from build123d import *

# Parameters (mm, degrees)
SKETCH2_W           = 15
SKETCH2_H           = 20
BOSS_EXTRUDE1_DEPTH = 9
SKETCH3_R           = 1.75
CUT_EXTRUDE1_DEPTH  = 18.400072003
SKETCH4_W           = 35
SKETCH4_H           = 15
BOSS_EXTRUDE2_DEPTH = 9
SKETCH5_R           = 1.75
CUT_EXTRUDE2_DEPTH  = 47.61728645


with BuildPart() as part:
    # Sketch2 → Boss-Extrude1 (new body)
    with BuildSketch(Plane(origin=(0, 0, 0), x_dir=(0, 0, -1), z_dir=(1, 0, 0))):
        with Locations((2.852361856, -0.704723711)):
            Rectangle(SKETCH2_W, SKETCH2_H)
    extrude(amount=BOSS_EXTRUDE1_DEPTH)

    # Sketch3 → Cut-Extrude1 (cut, through all)
    with BuildSketch(Plane(origin=(9, 0, 0), x_dir=(0, 0, -1), z_dir=(1, 0, 0))):
        with Locations((2.852361856, -5.704723711)):
            Circle(SKETCH3_R)
        with Locations((2.852361856, 4.295276289)):
            Circle(SKETCH3_R)
    extrude(amount=-CUT_EXTRUDE1_DEPTH, mode=Mode.SUBTRACT)

    # Sketch4 → Boss-Extrude2 (add)
    with BuildSketch(Plane(origin=(0, 9.295276289, 0), x_dir=(1, 0, 0), z_dir=(0, 1, 0))):
        with Locations((17.5, 2.852361856)):
            Rectangle(SKETCH4_W, SKETCH4_H)
    extrude(amount=BOSS_EXTRUDE2_DEPTH)

    # Sketch5 → Cut-Extrude2 (cut, through all)
    with BuildSketch(Plane(origin=(0, 18.295276289, 0), x_dir=(1, 0, 0), z_dir=(0, 1, 0))):
        with Locations(Location((12, 2.852361856, 0), (0, 0, 270))):
            Circle(SKETCH5_R)
        with Locations(Location((22, 2.852361856, 0), (0, 0, 270))):
            Circle(SKETCH5_R)
    extrude(amount=-CUT_EXTRUDE2_DEPTH, mode=Mode.SUBTRACT)


solid = part.part
Here's how the part is built. I have some questions about the finished solid (model axes, mm). A direction names the side the tool comes from. Coordinates: 2 decimals unless noted, no trailing zeros. Order: outer loops, then holes, each group sorted by start corner. A loop starts at its lowest first (then second) coordinate and runs counter-clockwise, first axis right, second up.
Item 1: If we section it at B-B on z = -9: List the corners of the cut face in (x, y) for me.
Result sheet:
outline: (0, -10.7) - (9, -10.7) - (9, 9.3) - (35, 9.3) - (35, 18.3) - (0, 18.3) - close
Item 2: If we section it at A-A on x = 22: List the corners of the cut face in (y, z) for me, plus the area to 4 significant figures.
Result sheet:
outline: (9.3, -10.35) - (18.3, -10.35) - (18.3, -4.6) - (9.3, -4.6) - close; (9.3, -1.1) - (18.3, -1.1) - (18.3, 4.65) - (9.3, 4.65) - close
area: 103.5 mm2
Item 3: For faces 1 (the face through (22, 9.295, -5)), 2 (the face through (23.735, 13.858, -3.08)), which set-ups out of +Z, -Z, +X, -X, +Y, -Y let a thin tool reach every point of the face, with its end or its side?
Result sheet:
face 1: +Z, -Z, +X, -Y
face 2: +Y, -Y
Item 4: If we mould it in two halves opening along Z, with no side actions, what happens to faces 3 (the face through (0, 3.59, -1.08)), 4 (the face through (13, 10, -10.352)), 5 (the face through (13, 10, 4.648)), 6 (the face through (4.56, 4.82, -4.52))? For each: +Z half, -Z half, draft (parallel to the pull), parting line (faces both ways), or undercut.
Result sheet:
face 3: draft
face 4: -Z half
face 5: +Z half
face 6: undercut
Item 5: If we section it at C-C on y = 15.75: List the corners of the cut face in (x, z) for me, plus the area to 3 significant figures.
Result sheet:
outline: (0, -10.35) - (35, -10.35) - (35, 4.65) - (0, 4.65) - close; hole circle Ø3.5 at (12, -2.85); hole circle Ø3.5 at (22, -2.85)
area: 506 mm2
Item 6: I need wall thicknesses on line 1 (X direction, y = 16, z = -3); line 2 (Y direction, x = 7, z = -4); line 3 (X direction, y = -7.5, z = -3). Which ranges of each line are inside material? Lowest first, please.
Result sheet:
line 1: x = 0 to 10.26, 13.74 to 20.26, 23.74 to 35
line 2: y = -10.7 to -7.03, -4.38 to 2.97, 5.62 to 18.3
line 3: x = 0 to 9
Item 7: For P1, Ø4.5, axis at y = 3.5, z = -4.5, coming from the +X side; P2, Ø5.5, axis at x = 22, z = -2.85, coming from the +Y side; P3, Ø4, axis at x = 17.5, z = 1, coming from the -Y side, each with a flat end and sliding along its axis, tell me the tip position at first contact or that it passes through.
Result sheet:
P1: stops at x = 9
P2: stops at y = 18.3
P3: stops at y = 9.3
